```python
from build123d import *


with BuildPart() as f1:
    # F0 (on Front) → F1 (revolve)
    with BuildSketch(Plane.XZ):
        with BuildLine():
            Line((24.85, 1.5), (28.35, 1.5))
            ThreePointArc((28.35, 1.5), (27.481033, 3.525), (28.35, 5.55))
            Line((28.35, 5.55), (24.85, 5.55))
            Line((24.85, 5.55), (24.85, 1.5))
        make_face()
        with BuildLine():
            Line((37.56, 0), (38.7, 0))
            Line((38.7, 0), (38.7, 7.05))
            Line((38.7, 7.05), (37.56, 7.05))
            Line((37.56, 7.05), (37.56, 5.55))
            Line((37.56, 5.55), (32.2, 5.55))
            ThreePointArc((32.2, 5.55), (32.842551, 4.626786), (33.068967, 3.525))
            ThreePointArc((33.068967, 3.525), (32.842551, 2.423214), (32.2, 1.5))
            Line((32.2, 1.5), (37.56, 1.5))
            Line((37.56, 1.5), (37.56, 0))
        make_face()
        with BuildLine():
            ThreePointArc((28.35, 1.5), (30.275, 0.731033), (32.2, 1.5))
            ThreePointArc((32.2, 1.5), (32.842551, 2.423214), (33.068967, 3.525))
            ThreePointArc((33.068967, 3.525), (32.842551, 4.626786), (32.2, 5.55))
            ThreePointArc((32.2, 5.55), (30.275, 6.318967), (28.35, 5.55))
            ThreePointArc((28.35, 5.55), (27.481033, 3.525), (28.35, 1.5))
        make_face()
    revolve(axis=Axis((0, 0, 3.525), (0, 0, 1)))


solid = f1.part
```
Read the model definition and answer for the solid it produces. Units are mm, in the model's axes. A direction names the side the tool comes from. Give positions to 0.01 mm unless a question says otherwise; leave off trailing zeros. Write each loop counter-clockwise with the first axis right and the second up, starting at its lowest first coordinate (ties: lowest second). Pieces come first, ordered by that corner, then holes. Notation, with made-up numbers: (-24, 29.5) - (7, 29.5) arc R16 cw to (7, 44.5) - close; hole circle Ø10 at (19.5, 68). An arc over 180 degrees is marked (long way). Write item = value, one per line. Start each with the question number.
Item 1: Find the intervals of material crossed by probe 1 along X at (y, z) = (1, 6.5); probe 2 along Y at (x, z) = (0, 6.65); probe 3 along Y at (x, z) = (0, 1.05), in increasing order. Write a range as [from, to].
Item 2: Each of these flat-tipped pins is pushed along its axis until it touches: P1, Ø2, axis at y = -7.5, z = 3, coming from the -X side; P2, Ø1.5, axis at y = 14.5, z = 6, coming from the +X side; P3, Ø12, axis at x = 12.5, y = -18, coming from the -Z side. Where does it stop, or does it pass through?
Item 3: Find section C-C (z = 3.25). Give the vertices of the cut face in (x, y).
Item 4: The mould has two halves that part along X. Classify faces 4 (the cylindrical face through (-38.663, 1.702, 3.574)), 5 (the cylindrical face through (-19.72, -15.12, 3.5)), 6 (the flat face through (-20, 32, 7.05)), 7 (the flat face through (-0.1, -25.1, 5.55)): +X half, -X half, draft (parallel to the pull), parting line (faces both ways), or undercut.
Item 5: A tool of negligible diameter and unlimited length cuts with its end or side. For faces 1 (the flat face through (20, 32, 0)), 2 (the cylindrical face through (-37.524, 1.651, 0.74)), 3 (the flat face through (28, 17, 5.55)), from which of +Z, -Z, +X, -X, +Y, -Y can it reach the whole face along a straight path? Write none if from no direction.
Item 6: Find section A-A (y = 0). Give the vertices of the cut face in (x, z) (3 decimals), then the cut area to 3 significant figures.
Response:
q1.probe_1 = [-38.69, -37.55], [37.55, 38.69]
q1.probe_2 = [-38.7, -37.56], [37.56, 38.7]
q1.probe_3 = [-38.7, -37.56], [-31.57, -28.98], [28.98, 31.57], [37.56, 38.7]
q2.P1 = -38.15
q2.P2 = 36.17
q2.P3 = 1.5
q3.outline = circle Ø77.4 at (0, 0); hole circle Ø49.7 at (0, 0)
q4.face_4 = parting line
q4.face_5 = undercut
q4.face_6 = draft
q4.face_7 = undercut
q5.face_1 = -Z, +X, -X, +Y, -Y
q5.face_2 = -Z
q5.face_3 = +Z
q6.outline = (-38.7, 0) - (-37.56, 0) - (-37.56, 1.5) - (-32.2, 1.5) arc R2.794 ccw to (-28.35, 1.5) - (-24.85, 1.5) - (-24.85, 5.55) - (-28.35, 5.55) arc R2.794 ccw to (-32.2, 5.55) - (-37.56, 5.55) - (-37.56, 7.05) - (-38.7, 7.05) - close; (24.85, 1.5) - (28.35, 1.5) arc R2.794 ccw to (32.2, 1.5) - (37.56, 1.5) - (37.56, 0) - (38.7, 0) - (38.7, 7.05) - (37.56, 7.05) - (37.56, 5.55) - (32.2, 5.55) arc R2.794 ccw to (28.35, 5.55) - (24.85, 5.55) - close
q6.area = 127 mm²
